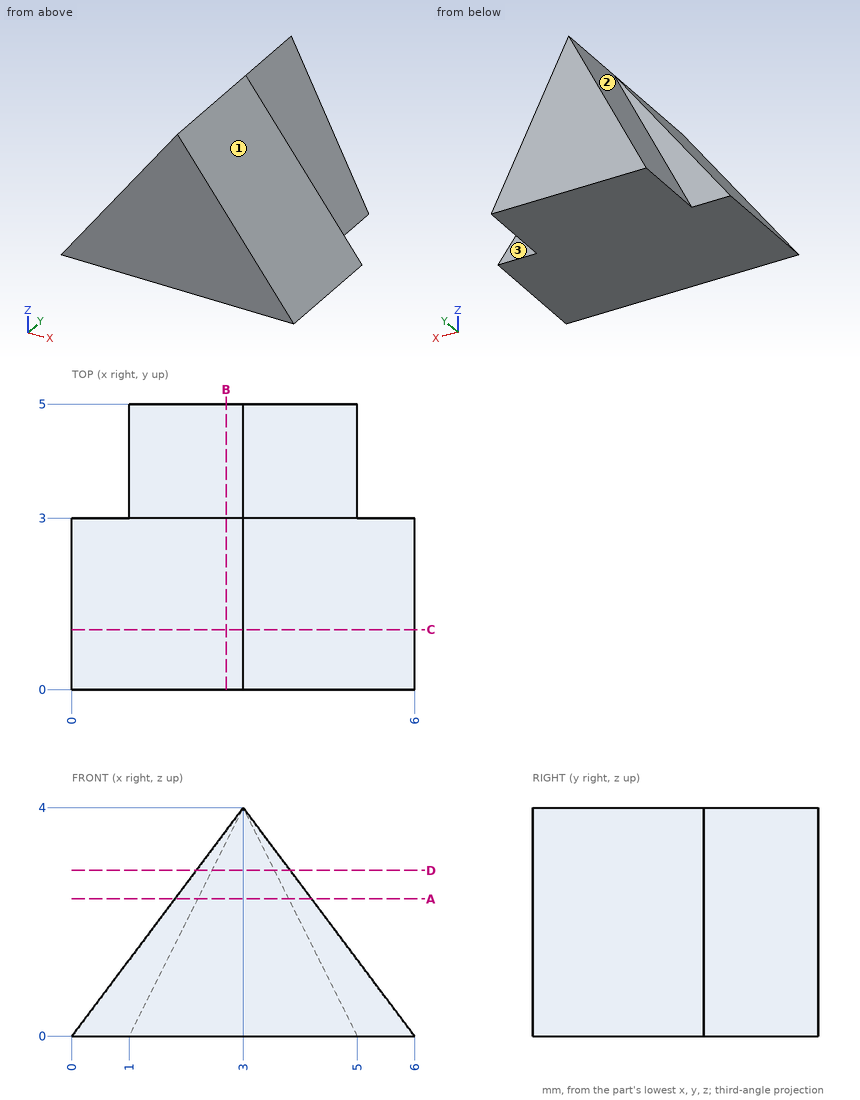
Geometry: see drawing. Coordinates: mm, zero at the bounding-box minimum. A direction names the side the tool comes from. Round coordinates to 2 decimals unless told otherwise and drop trailing zeros. Write each loop counter-clockwise with the first axis right and the second up, starting at its lowest first coordinate (ties: lowest second). Pieces come first, ordered by that corner, then holes. Notation, with made-up numbers: M 60.25,3.25 L 116.25,3.25 A6 cw 116.25,7.25 Z; hole C -28.75,-22 d5. An arc over 180 degrees is marked long. Answer in a Markdown table with one row per item. Add a question column.
(1) Ray query, L1, parallel to Z at x = 2.5, y = 3.8; L2, parallel to Z at x = 4.7, y = 0.3; L3, parallel to X at y = 1.4, z = 0.4. Return the intervals inside material, ascending.
(2) Cut plane B-B, the plane x = 2.7. Return the cut outline in (y, z), then the cut area to 3 significant figures.
(3) Cut plane D-D, the plane z = 2.9. Return the cut outline in (x, y) (3 decimals), then the cut area to 3 significant figures.
(4) Cut plane C-C, the plane y = 1.05. Return the cut outline in (x, z), then the cut area to 3 significant figures.
(5) Reachability of the marked faces 1, 2 and 3 from +Z, -Z, +X, -X, +Y, -Y: full face, straight path, thin tool, end or side. Return the list, or none.
(6) Cut plane A-A, the plane z = 2.4. Return the cut outline in (x, y), then the cut area to 3 significant figures.
(7) Contact query for flat-ended pins moving along their axis: pin 1 (1 mm diameter, centred on y = 0.5, z = 2.5, fed in from +X); pin 2 (1 mm diameter, centred on y = 1.5, z = 3, fed in from +X) (3 decimals); pin 3 (1 mm diameter, centred on y = 2.5, z = 3, fed in from -X) (3 decimals). Output: stop coordinate, or through.
Established:
| question | item | result |
|---|---|---|
| 1 | L1 | 0 to 3 |
| 1 | L2 | 0 to 1.73 |
| 1 | L3 | 0.3 to 5.7 |
| 2 | outline | M 0,0 L 5,0 L 5,3.4 L 3,3.4 L 3,3.6 L 0,3.6 Z |
| 2 | area | 17.6 mm² |
| 3 | outline | M 2.175,0 L 3.825,0 L 3.825,3 L 3.55,3 L 3.55,5 L 2.45,5 L 2.45,3 L 2.175,3 Z |
| 3 | area | 7.15 mm² |
| 4 | outline | M 0,0 L 6,0 L 3,4 Z |
| 4 | area | 12.0 mm² |
| 5 | face 1 | +Z, +X, +Y, -Y |
| 5 | face 2 | +Z, -X, +Y |
| 5 | face 3 | +Z, +X, +Y |
| 6 | outline | M 1.8,0 L 4.2,0 L 4.2,3 L 3.8,3 L 3.8,5 L 2.2,5 L 2.2,3 L 1.8,3 Z |
| 6 | area | 10.4 mm² |
| 7 | pin 1 | x = 4.5 |
| 7 | pin 2 | x = 4.125 |
| 7 | pin 3 | x = 1.875 |
